Can you work these out from the model? Positions are in its coordinate system, mm. Face numbers are marked on the shaded views. A direction names the side the tool comes from. Round coordinates to 2 decimals unless told otherwise and drop trailing zeros. Order: outer loops, then holes, each group sorted by start corner. A loop starts at its lowest first (then second) coordinate and runs counter-clockwise, first axis right, second up. Notation, with made-up numbers: M 29.5,-1.5 L 59.5,-1.5 A27 ccw 59.5,23.5 Z; hole C 71,-37.5 d11. An arc over 180 degrees is marked long. One line per question, with ' | ' between items.
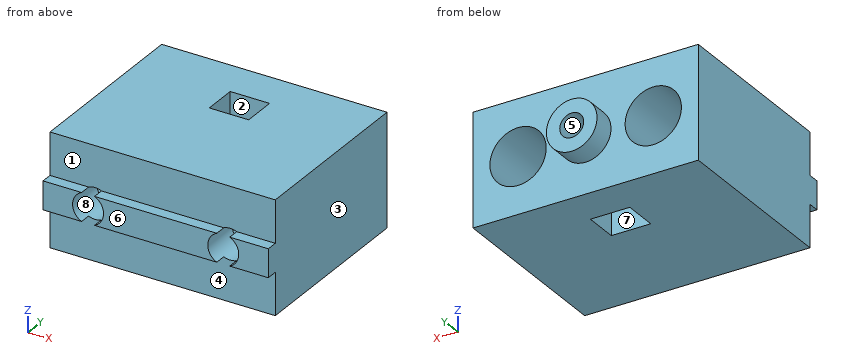
```python
from build123d import *

# Parameters (mm, degrees)
SKETCH1_W           = 40
SKETCH1_H           = 20
BOSS_EXTRUDE1_DEPTH = 32
SKETCH2_W           = 40
SKETCH2_H           = 5
BOSS_EXTRUDE2_DEPTH = 2
SKETCH3_R           = 2.75
CUT_EXTRUDE1_DEPTH  = 35
SKETCH4_R           = 5
CUT_EXTRUDE2_DEPTH  = 27
SKETCH5_W           = 7
SKETCH5_H           = 6
CUT_EXTRUDE3_DEPTH  = 21
SKETCH6_R           = 4.5
BOSS_EXTRUDE3_DEPTH = 4
SKETCH7_R           = 2.125
CUT_EXTRUDE4_DEPTH  = 20


with BuildPart() as part:
    # Sketch1 → Boss-Extrude1 (new body)
    with BuildSketch(Plane(origin=(0, 0, 0), x_dir=(1, 0, 0), z_dir=(0, 1, 0))):
        with Locations((20, 10)):
            Rectangle(SKETCH1_W, SKETCH1_H)
    extrude(amount=BOSS_EXTRUDE1_DEPTH)

    # Sketch2 → Boss-Extrude2 (add)
    with BuildSketch(Plane.XZ):
        with Locations((20, -10)):
            Rectangle(SKETCH2_W, SKETCH2_H)
    extrude(amount=BOSS_EXTRUDE2_DEPTH)

    # Sketch3 → Cut-Extrude1 (cut, through all)
    with BuildSketch(Plane(origin=(0, 32, 0), x_dir=(1, 0, 0), z_dir=(0, 1, 0))):
        with Locations((32, 10)):
            Circle(SKETCH3_R)
        with Locations((8, 10)):
            Circle(SKETCH3_R)
    extrude(amount=-CUT_EXTRUDE1_DEPTH, mode=Mode.SUBTRACT)

    # Sketch4 → Cut-Extrude2 (cut)
    with BuildSketch(Plane(origin=(0, 32, 0), x_dir=(1, 0, 0), z_dir=(0, 1, 0))):
        with Locations((8, 10)):
            Circle(SKETCH4_R)
        with Locations((32, 10)):
            Circle(SKETCH4_R)
    extrude(amount=-CUT_EXTRUDE2_DEPTH, mode=Mode.SUBTRACT)

    # Sketch5 → Cut-Extrude3 (cut, through all)
    with BuildSketch(Plane.XY):
        with Locations((20, 22)):
            Rectangle(SKETCH5_W, SKETCH5_H)
    extrude(amount=-CUT_EXTRUDE3_DEPTH, mode=Mode.SUBTRACT)

    # Sketch6 → Boss-Extrude3 (add)
    with BuildSketch(Plane(origin=(0, 32, 0), x_dir=(1, 0, 0), z_dir=(0, 1, 0))):
        with Locations((20, 10)):
            Circle(SKETCH6_R)
    extrude(amount=BOSS_EXTRUDE3_DEPTH)

    # Sketch7 → Cut-Extrude4 (cut)
    with BuildSketch(Plane(origin=(0, 36, 0), x_dir=(1, 0, 0), z_dir=(0, 1, 0))):
        with Locations((20, 10)):
            Circle(SKETCH7_R)
    extrude(amount=-CUT_EXTRUDE4_DEPTH, mode=Mode.SUBTRACT)


solid = part.part
```
(1) Will these pins go through, and if not, where does the flat tip stop? pin 1 Ø1 at (x, y) = (37.5, -1) entering from -Z; pin 2 Ø4 at (x, z) = (30.5, -11.5) entering from +Y; pin 3 Ø8 at (x, z) = (10, -15) entering from +Y.
Final values:
pin 1: z = -12.5 | pin 2: y = 5 | pin 3: y = 32
(2) If we section it at B-B on z = -1.5: Please give me the cut outline in (x, y).
Final values:
outline: M 0,0 L 40,0 L 40,32 L 0,32 Z; hole M 16.5,19 L 23.5,19 L 23.5,25 L 16.5,25 Z
(3) Thinking about a two-plate mould opening in Y: for the marked faces 6, 7 and 8, which applies, released by +Y, released by -Y, zero draft, split by the parting line, or undercut?
Final values:
face 6: released by -Y | face 7: undercut | face 8: zero draft
(4) If we section it at A-A on x = 32: Please give me the cut outline in (y, z), plus the area to 4 significant figures.
Final values:
outline: M 0,-20 L 32,-20 L 32,-15 L 5,-15 L 5,-12.75 L 0,-12.75 Z; M 0,-7.25 L 5,-7.25 L 5,-5 L 32,-5 L 32,0 L 0,0 Z | area: 342.5 mm^2
(5) If we section it at C-C on x = 20: Please give me the cut outline in (y, z) (3 decimals), plus the area to 4 significant figures.
Final values:
outline: M -2,-12.5 L 0,-12.5 L 0,-20 L 19,-20 L 19,-12.125 L 16,-12.125 L 16,-7.875 L 19,-7.875 L 19,0 L 0,0 L 0,-7.5 L -2,-7.5 Z; M 25,-20 L 32,-20 L 32,-14.5 L 36,-14.5 L 36,-12.125 L 25,-12.125 Z; M 25,-7.875 L 36,-7.875 L 36,-5.5 L 32,-5.5 L 32,0 L 25,0 Z | area: 506.5 mm^2
(6) On a 3-axis mill with a long thin cutter (end or side, diameter ignored), from which of +Z, -Z, +X, -X, +Y, -Y can I reach the whole of each face in a straight line? I mean the marked faces 1, 2, 3, 4 and 5. Say none if no direction works.
Final values:
face 1: +Z, +X, -X, -Y | face 2: +Z, -Z | face 3: +Z, -Z, +X, +Y, -Y | face 4: -Z, +X, -X, -Y | face 5: +Y
(7) Please list where these lines run through material, in increasing order: probe 1 along X at (y, z) = (17.65, -10) (3 decimals); probe 2 along X at (y, z) = (2, -10); probe 3 along X at (y, z) = (24, -10). Write a range as [from, to].
Final values:
probe 1: [0, 3], [13, 17.875], [22.125, 27], [37, 40] | probe 2: [0, 5.25], [10.75, 29.25], [34.75, 40] | probe 3: [0, 3], [13, 16.5], [23.5, 27], [37, 40]
(8) If we section it at D-D on y = 31: Please give me the cut outline in (x, z) (3 decimals), plus the area to 3 significant figures.
Final values:
outline: M 0,-20 L 40,-20 L 40,0 L 0,0 Z; hole C 8,-10 d10; hole C 20,-10 d4.25; hole C 32,-10 d10 | area: 629 mm^2
